Design review of the part built by this model. Coordinates are the model's own, in mm. Coordinates: 2 decimals unless noted, no trailing zeros. Loops run counter-clockwise (first coordinate to the right, second up) from the corner with the lowest first, then second, coordinate; pieces in that order, holes last. Notation, with made-up numbers: (34.5, 82) - (54.5, 82) arc R25 ccw to (54.5, 116) - close; hole circle Ø5 at (42.25, 16). An arc over 180 degrees is marked (long way). Return JSON: item names as keys, results as strings. Group by question number.
Autodesk Inventor part; units mm, degrees
ref_plane "YZ Plane" through (0, 0, 0) normal (1, 0, 0) x (0, 1, 0)
ref_plane "XZ Plane" through (0, 0, 0) normal (0, 1, 0) x (-1, 0, 0)
ref_plane "XY Plane" through (0, 0, 0) normal (0, 0, 1) x (1, 0, 0)
sketch "Sketch1" plane through (0, 0, 0) normal (0, 1, 0) x (-1, 0, 0)
  line L0 (101.6, 38.1) -> (-101.6, 38.1) construction
  line L1 (-101.6, 38.1) -> (-101.6, -38.1) construction
  line L2 (-101.6, -38.1) -> (101.6, -38.1) construction
  line L3 (101.6, -38.1) -> (101.6, 38.1) construction
  line L4 (101.6, 38.1) -> (-101.6, -38.1) construction
  line L5 (-101.6, 38.1) -> (101.6, -38.1) construction
  line L6 (-28.575, 66.675) -> (28.575, 66.675) construction
  line L7 (28.575, 66.675) -> (28.575, 9.525) construction
  line L8 (28.575, 9.525) -> (-28.575, 9.525)
  line L9 (-28.575, 9.525) -> (-28.575, 66.675) construction
  line L10 (-28.575, 66.675) -> (28.575, 9.525) construction
  line L11 (28.575, 66.675) -> (-28.575, 9.525) construction
  circle A0 centre (-38.1, 50.8) radius 3.175 construction
  line L12 (0, 38.1) -> (0, -38.1) construction
  circle A1 centre (-38.1, 50.8) radius 9.525 construction
  line L13 (-38.1, 60.325) -> (-28.575, 60.325) construction
  circle A2 centre (38.1, 50.8) radius 3.175 construction
  circle A3 centre (38.1, 50.8) radius 9.525 construction
  line L14 (38.1, 60.325) -> (28.575, 60.325) construction
  circle A4 centre (-76.2, -38.1) radius 1.7526 construction
  circle A5 centre (-95.25, 3.175) radius 1.7526 construction
  circle A6 centre (76.2, -38.1) radius 1.7526 construction
  circle A7 centre (95.25, 3.175) radius 1.7526 construction
  line L15 (-101.6, -38.1) -> (-101.6, 6.35) construction
  line L16 (-101.6, 6.35) -> (-44.4797, 57.8728) construction
  line L17 (101.6, -38.1) -> (101.6, 6.35) construction
  line L18 (101.6, 6.35) -> (44.4797, 57.8728) construction
  line L19 (-42.6417, 42.4275) -> (-87.975, 1.5367) construction
  line L20 (-87.975, 1.5367) -> (-87.975, -38.1) construction
  line L21 (87.975, -38.1) -> (87.975, 1.5367) construction
  line L22 (87.975, 1.5367) -> (42.6417, 42.4275) construction
  line L23 (0, -38.1) -> (-95.25, -38.1) construction
  line L24 (0, -38.1) -> (95.25, -38.1) construction
  circle A8 centre (-60.325, 35.0287) radius 1.7526 construction
  circle A9 centre (-33.3375, 31.75) radius 1.7526 construction
  line L25 (-38.1, 0) -> (-38.1, 41.275) construction
  line L26 (-38.1, 0) -> (0, 0) construction
  circle A10 centre (60.325, 35.0287) radius 1.7526 construction
  circle A11 centre (33.3375, 31.75) radius 1.7526 construction
  line L27 (38.1, 0) -> (38.1, 41.275) construction
  line L28 (38.1, 0) -> (0, 0) construction
  line L29 (-87.975, 0) -> (-65.115, 0) construction
  line L30 (-65.115, 0) -> (-65.115, -31.75) construction
  line L31 (-65.115, -31.75) -> (-87.975, -31.75) construction
  line L32 (-101.6, -38.1) -> (101.6, -38.1) construction
  line L33 (101.6, -38.1) -> (101.6, 19.05) construction
  line L34 (101.6, 19.05) -> (-101.6, 19.05) construction
  line L35 (-101.6, 19.05) -> (-101.6, -38.1) construction
  line L36 (-101.6, 19.05) -> (-87.5203, 19.05) construction
  line L37 (87.5203, 19.05) -> (101.6, 19.05) construction
  circle A12 centre (-38.1, 0) radius 3.175 construction
  circle A13 centre (-38.1, 0) radius 6.35 construction
  circle A14 centre (38.1, 0) radius 3.175 construction
  circle A15 centre (38.1, 0) radius 6.35 construction
  circle A16 centre (28.575, 9.525) radius 1.7526
  circle A17 centre (28.575, 9.525) radius 4.7625
  arc A18 (17.0773, 9.525) -> (28.575, 21.0227) centre (17.0773, 21.0227) ccw
  circle A19 centre (-28.575, 9.525) radius 1.7526
  circle A20 centre (-28.575, 9.525) radius 4.7625
  arc A21 (-28.575, 21.0227) -> (-17.0773, 9.525) centre (-17.0773, 21.0227) ccw
  arc A22 (31.4325, 5.715) -> (38.1, 19.05) centre (21.4312, 19.05) ccw construction
  arc A23 (-38.1, 19.05) -> (-31.4325, 5.715) centre (-21.4312, 19.05) ccw construction
  line L38 (-61.94, -38.1) -> (-61.94, 25.0204) construction
  line L39 (87.975, 0) -> (65.115, 0) construction
  line L40 (65.115, 0) -> (65.115, -31.75) construction
  line L41 (65.115, -31.75) -> (87.975, -31.75) construction
  line L42 (61.94, -38.1) -> (61.94, 25.0204) construction
  line L43 (-28.575, 4.7625) -> (28.575, 4.7625) construction
  line L44 (101.6, -31.75) -> (-101.6, -31.75) construction
  line L45 (-101.6, -31.75) -> (-101.6, -44.45) construction
  line L46 (-101.6, -44.45) -> (101.6, -44.45)
  line L47 (101.6, -44.45) -> (101.6, -31.75) construction
  circle A24 centre (0, -38.1) radius 1.7526
  circle A25 centre (38.1, -38.1) radius 1.7526
  circle A26 centre (-38.1, -38.1) radius 1.7526
  line L48 (101.6, -38.1) -> (76.2, -44.45) construction
  line L49 (-101.6, -38.1) -> (-76.2, -44.45) construction
  line L50 (76.2, -38.1) -> (76.2, -44.45) construction
  line L51 (-76.2, -38.1) -> (-76.2, -44.45) construction
  line L52 (59.1924, 41.2769) -> (32.488, 36.4361) construction
  circle A27 centre (60.325, 35.0287) radius 6.35 construction
  circle A28 centre (33.3375, 31.75) radius 4.7625 construction
  line L53 (-59.1924, 41.2769) -> (-32.488, 36.4361) construction
  circle A29 centre (-60.325, 35.0287) radius 6.35 construction
  circle A30 centre (-33.3375, 31.75) radius 4.7625 construction
  line L54 (-87.975, 0) -> (-65.115, 0) construction
  line L55 (-65.115, 0) -> (-65.115, -3.175) construction
  line L56 (-65.115, -3.175) -> (-87.975, -3.175) construction
  line L57 (-87.975, -3.175) -> (-87.975, 0) construction
  line L58 (-65.115, -15.875) -> (-87.975, -15.875) construction
  line L59 (-65.115, -28.575) -> (-87.975, -28.575) construction
  line L60 (-84.8, -38.1) -> (-84.8, 0.1248) construction
  line L61 (65.115, -3.175) -> (87.975, -3.175) construction
  line L62 (65.115, -15.875) -> (87.975, -15.875) construction
  line L63 (65.115, -28.575) -> (87.975, -28.575) construction
  line L64 (84.8, -38.1) -> (84.8, 0.1248) construction
  line L65 (-31.75, -31.75) -> (31.75, -31.75) construction
  line L66 (31.75, -31.75) -> (31.75, 0) construction
  line L67 (31.75, 0) -> (-31.75, 0) construction
  line L68 (-31.75, 0) -> (-31.75, -31.75) construction
  circle A31 centre (71.465, 12.7) radius 3.175 construction
  circle A32 centre (-71.465, 12.7) radius 3.175 construction
  circle A33 centre (38.1, -38.1) radius 6.35
  circle A34 centre (-38.1, -38.1) radius 6.35
  line L69 (44.2827, -36.6518) -> (33.212, 10.6111)
  line L70 (-44.2827, -36.6518) -> (-33.212, 10.6111)
  point P0 (28.575, 38.1)
  point P1 (-28.575, 38.1)
  point P2 (28.575, 60.325)
  point P3 (44.4797, 57.8728)
  point P4 (101.6, -15.875)
  point P5 (38.1, 41.275)
  point P6 (-87.975, -31.75)
  point P7 (-101.6, 6.35)
  point P8 (101.6, 6.35)
  point P9 (31.75, 0)
  point P10 (38.1, 6.35)
  point P11 (-38.1, 6.35)
  point P12 (-31.75, 0)
  point P13 (87.975, 0)
  point P14 (61.94, 25.0204)
  point P15 (-17.0773, 9.525)
  point P16 (-28.575, 21.0227)
  point P17 (-38.1, 19.05)
  point P18 (-31.4325, 5.715)
  point P19 (-21.8502, 0)
  point P20 (21.8502, 0)
  point P21 (-25.2074, 12.8926)
  point P22 (-28.575, 14.2875)
  point P23 (-23.8125, 9.525)
  point P24 (-28.575, 50.8)
  point P25 (25.2074, 12.8926)
  point P26 (28.575, 14.2875)
  point P27 (23.8125, 9.525)
  point P28 (28.575, 50.8)
  point P29 (26.8224, 9.525)
  point P30 (28.575, 11.2776)
  point P31 (61.94, -31.75)
  point P32 (-61.94, -31.75)
  point P33 (-28.575, 31.75)
  point P34 (-64.5781, 39.7439)
  point P35 (64.5781, 39.7439)
  point P36 (28.575, 31.75)
  point P37 (-84.8, -3.175)
  point P38 (-84.8, -28.575)
  point P39 (84.8, -3.175)
  point P40 (84.8, -28.575)
  point P41 (31.75, -31.75)
  point P42 (-101.6, -31.75)
  point P43 (31.75, -31.75)
  point P44 (-26.8224, 9.525)
  point P45 (-28.575, 11.2776)
  point P46 (-39.8526, -38.1)
  point P47 (-36.3474, -38.1)
  point P48 (-1.7526, -38.1)
  point P49 (1.7526, -38.1)
  point P50 (36.3474, -38.1)
  point P51 (39.8526, -38.1)
  point P52 (-38.1, -44.45)
  point P53 (38.1, -44.45)
  dimension "d0" = 203.2
  dimension "d1" = 76.2
  dimension "d4" = 57.15
  dimension "d6" = 6.35
  dimension "d7" = 38.1
  dimension "d8" = 19.05
  dimension "d10" = 3.5052
  dimension "d11" = 3.5052
  dimension "d12" = 0
  dimension "d14" = 25.4
  dimension "d15" = 6.35
  dimension "d20" = 50.8
  dimension "d21" = 41.275
  dimension "d22" = 44.45
  dimension "d24" = 12.7
  dimension "d25" = 13.625
  dimension "d26" = 12.7
  dimension "d27" = 13.625
  dimension "d31" = 3.5052
  dimension "d32" = 3.5052
  dimension "d33" = 6.35
  dimension "d34" = 31.75
  dimension "d35" = 4.7625
  dimension "d36" = 22.225
  dimension "d37" = 9.525
  dimension "d39" = 31.75
  dimension "d40" = 6.35
  dimension "d42" = 57.15
  dimension "d43" = 6.35
  dimension "d44" = 9.525
  dimension "d45" = 9.525
  dimension "d46" = 12.7
  dimension "d104" = 3.5052
  dimension "d105" = 9.525
  dimension "d106" = 3.175
  dimension "d107" = 22.86
  dimension "d123" = 88.9
  dimension "d124" = 12.7
  dimension "d125" = 3.5052
  dimension "d126" = 3.5052
  dimension "d127" = 38.1
  dimension "d128" = 28.575
  dimension "d129" = 3.175
  dimension "d130" = 3.175
  dimension "d131" = 31.75
  dimension "d132" = 31.75
  dimension "d133" = 31.75
  dimension "d135" = 6.35
  dimension "d136" = 12.7
  dimension "d137" = 9.525
extrude "Extrusion1" add sketch "Sketch1" along normal blind 3.175
equation "\"d35\" = 0.5 * d37"
properties part number "Chassis" material "UHMW, White"
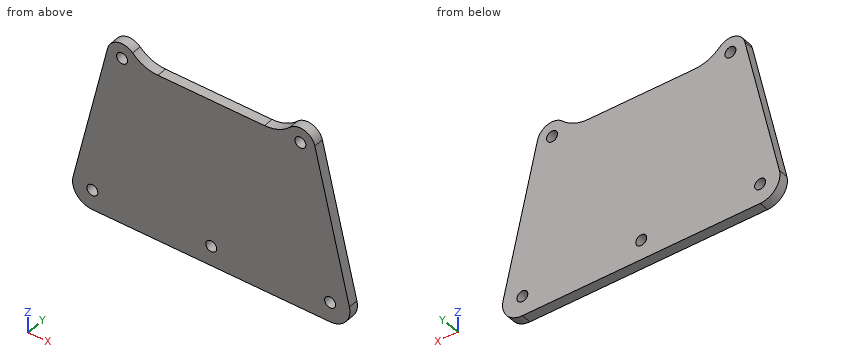
Item 1: Add section D-D (x = -12). State the section outline as (y, z) points (3 decimals).
Item 2: Add section B-B (z = -38.1). State the section outline as (x, y) points (3 decimals), then the cut area to 3 significant figures.
Item 3: Add section A-A (x = 0). State the section outline as (y, z) points (3 decimals), then the cut area to 3 significant figures.
Item 4: To check wall thickness, follow line 1 (X direction, y = 1.1, z = -37); line 2 (Z direction, x = 0, y = 1.6) (3 decimals); line 3 (Z direction, x = -6, y = 2.15) (3 decimals). State the ranges of each line that lie inside material, in increasing order. Write a range as from..to.
Item 5: Add section C-C (y = 2.5). Give the number of separate pieces and of enclosed holes in the cut face, then the cut area to 3 significant figures.
Item 6: For P1, Ø3, axis at x = 38.1, z = -38.1, coming from the -Y side; P2, Ø1, axis at y = 1.5, z = -6, coming from the -X side, all flat-tipped, find the tip position at first contact; note any pin that passes through.
Answers below:
{
 "1": {"outline": "(0, -44.45) - (3.175, -44.45) - (3.175, 9.525) - (0, 9.525) - close"},
 "2": {"outline": "(-44.45, 0) - (-39.853, 0) - (-39.853, 3.175) - (-44.45, 3.175) - close; (-36.347, 0) - (-1.753, 0) - (-1.753, 3.175) - (-36.347, 3.175) - close; (1.753, 0) - (36.347, 0) - (36.347, 3.175) - (1.753, 3.175) - close; (39.853, 0) - (44.45, 0) - (44.45, 3.175) - (39.853, 3.175) - close", "area": "249 mm^2"},
 "3": {"outline": "(0, -44.45) - (3.175, -44.45) - (3.175, -39.853) - (0, -39.853) - close; (0, -36.347) - (3.175, -36.347) - (3.175, 9.525) - (0, 9.525) - close", "area": "160 mm^2"},
 "4": {"line 1": "x = -44.35..-39.46, -36.74..-1.36, 1.36..36.74, 39.46..44.35", "line 2": "z = -44.45..-39.853, -36.347..9.525", "line 3": "z = -44.45..9.525"},
 "5": {"separate pieces": "1", "enclosed holes": "5", "area": "4,300 mm^2"},
 "6": {"P1": "passes through", "P2": "stops at x = -37.22"}
}
